```python
from build123d import *

# Parameters (mm, degrees)
Y_KSEKLIK_EKSTR_ZYON5_DEPTH      = 5
Y_KSEKLIK_EKSTR_ZYON5_DEPTH_BACK = 5
IZIM1_R                          = 37
IZIM1_R_2                        = 35.75
Y_KSEKLIK_EKSTR_ZYON6_DEPTH      = 3
Y_KSEKLIK_EKSTR_ZYON6_DEPTH_BACK = 3
IZIM1_13_R                       = 38.25
IZIM1_13_R_2                     = 37
Y_KSEKLIK_EKSTR_ZYON7_DEPTH      = 3
Y_KSEKLIK_EKSTR_ZYON7_DEPTH_BACK = 3
IZIM1_14_R                       = 1.5
Y_KSEKLIK_EKSTR_ZYON8_DEPTH      = 7
Y_KSEKLIK_EKSTR_ZYON8_DEPTH_BACK = 3


with BuildPart() as part:
    # Çizim1 → Yükseklik-Ekstrüzyon5 (new, two sides: drawn at the far end of the back side and taken through both)
    with BuildSketch(Plane.XY.offset(-Y_KSEKLIK_EKSTR_ZYON5_DEPTH_BACK)):
        Circle(IZIM1_R)
        Circle(IZIM1_R_2, mode=Mode.SUBTRACT)
    extrude(amount=Y_KSEKLIK_EKSTR_ZYON5_DEPTH + Y_KSEKLIK_EKSTR_ZYON5_DEPTH_BACK)

    # Çizim1<13> → Yükseklik-Ekstrüzyon6 (add, two sides: drawn at the far end of the back side and taken through both)
    with BuildSketch(Plane.XY.offset(-Y_KSEKLIK_EKSTR_ZYON6_DEPTH_BACK)):
        Circle(IZIM1_13_R)
        Circle(IZIM1_13_R_2, mode=Mode.SUBTRACT)
    extrude(amount=Y_KSEKLIK_EKSTR_ZYON6_DEPTH + Y_KSEKLIK_EKSTR_ZYON6_DEPTH_BACK)

    # Çizim1<14> → Yükseklik-Ekstrüzyon7 (add, two sides: drawn at the far end of the back side and taken through both)
    with BuildSketch(Plane.XY.offset(-Y_KSEKLIK_EKSTR_ZYON7_DEPTH_BACK)):
        with BuildLine():
            Line((0.352105211, 10.658426892), (0.352105211, 8.25))
            Line((0.352105211, 8.25), (0.352105211, 2.891667151))
            ThreePointArc((0.352105211, 2.891667151), (2.180757714, 1.931324101), (2.913025402, 0))
            ThreePointArc((2.913025402, 0), (-1.931880518, -2.180264813), (-0.350629391, 2.891846473))
            Line((-0.350629391, 2.891846473), (-0.347894744, 8.250178624))
            Line((-0.347894744, 8.250178624), (-0.346665593, 10.658605202))
            ThreePointArc((-0.346665593, 10.658605202), (-1.792646187, 11.069293289), (-2.984941087, 11.98469345))
            Line((-2.984941087, 11.98469345), (-14.607887345, 30.4259885))
            Line((-14.607887345, 30.4259885), (-14.847868654, 30.886461313))
            ThreePointArc((-14.847868654, 30.886461313), (-14.727142284, 32.060689053), (-13.92488883, 32.926584565))
            ThreePointArc((-13.92488883, 32.926584565), (-17.875, 30.960408185), (-21.552814278, 28.522599754))
            ThreePointArc((-21.552814278, 28.522599754), (-20.401800041, 28.78442387), (-19.324525803, 28.301862102))
            Line((-19.324525803, 28.301862102), (-19.045735303, 27.863795787))
            Line((-19.045735303, 27.863795787), (-8.886868167, 8.577081355))
            ThreePointArc((-8.886868167, 8.577081355), (-9.303777514, 5.496482546), (-11.800782256, 3.644761794))
            Line((-11.800782256, 3.644761794), (-33.653555768, 2.549643924))
            Line((-33.653555768, 2.549643924), (-34.19029782, 2.590308308))
            ThreePointArc((-34.19029782, 2.590308308), (-35.134400226, 3.283913251), (-35.477703108, 4.403984811))
            ThreePointArc((-35.477703108, 4.403984811), (-35.75, 0), (-35.477703108, -4.403984811))
            ThreePointArc((-35.477703108, -4.403984811), (-35.134400226, -3.283913251), (-34.19029782, -2.590308308))
            Line((-34.19029782, -2.590308308), (-33.653555768, -2.549643924))
            Line((-33.653555768, -2.549643924), (-11.802585687, -3.638917628))
            ThreePointArc((-11.802585687, -3.638917628), (-9.303458853, -5.492132995), (-8.888309481, -8.575587733))
            Line((-8.888309481, -8.575587733), (-19.045735303, -27.863795787))
            ThreePointArc((-19.045735303, -27.863795787), (-20.165883221, -28.700819486), (-21.552814278, -28.522599754))
            ThreePointArc((-21.552814278, -28.522599754), (-17.875, -30.960408185), (-13.92488883, -32.926584565))
            ThreePointArc((-13.92488883, -32.926584565), (-14.772697173, -31.814576902), (-14.607887345, -30.4259885))
            Line((-14.607887345, -30.4259885), (-2.984941087, -11.98469345))
            ThreePointArc((-2.984941087, -11.98469345), (0.002715908, -10.643228062), (2.991057136, -11.983168513))
            Line((2.991057136, -11.983168513), (14.663708375, -30.397995932))
            ThreePointArc((14.663708375, -30.397995932), (14.817986455, -31.815304786), (13.92488883, -32.926584565))
            ThreePointArc((13.92488883, -32.926584565), (17.875, -30.960408185), (21.552814278, -28.522599754))
            ThreePointArc((21.552814278, -28.522599754), (20.242255546, -28.76161283), (19.107217792, -28.064202809))
            Line((19.107217792, -28.064202809), (18.993975038, -27.89787469))
            Line((18.993975038, -27.89787469), (8.881942007, -8.582182507))
            ThreePointArc((8.881942007, -8.582182507), (9.294710999, -5.488602486), (11.804336715, -3.633233425))
            Line((11.804336715, -3.633233425), (33.657290889, -2.499854))
            Line((33.657290889, -2.499854), (33.849149755, -2.514104082))
            ThreePointArc((33.849149755, -2.514104082), (35.026532395, -3.146147751), (35.477703108, -4.403984811))
            ThreePointArc((35.477703108, -4.403984811), (35.681860841, -2.206197397), (35.75, 0))
            ThreePointArc((35.75, 0), (35.681860841, 2.206197397), (35.477703108, 4.403984811))
            ThreePointArc((35.477703108, 4.403984811), (35.026532395, 3.146147751), (33.849149755, 2.514104082))
            Line((33.849149755, 2.514104082), (33.657290889, 2.499854))
            Line((33.657290889, 2.499854), (11.803877394, 3.634725418))
            ThreePointArc((11.803877394, 3.634725418), (9.295867667, 5.489285508), (8.88302669, 8.581059795))
            Line((8.88302669, 8.581059795), (18.993975038, 27.89787469))
            Line((18.993975038, 27.89787469), (18.993582514, 27.898141932))
            ThreePointArc((18.993582514, 27.898141932), (20.143868947, 28.740405096), (21.552814278, 28.522599754))
            ThreePointArc((21.552814278, 28.522599754), (17.875, 30.960408185), (13.92488883, 32.926584565))
            ThreePointArc((13.92488883, 32.926584565), (14.817986455, 31.815304786), (14.663708375, 30.397995932))
            Line((14.663708375, 30.397995932), (14.663280674, 30.398202247))
            Line((14.663280674, 30.398202247), (2.991057136, 11.983168513))
            ThreePointArc((2.991057136, 11.983168513), (1.798295213, 11.068376963), (0.352105211, 10.658426892))
        make_face()
        with BuildLine():
            ThreePointArc((-15.330091906, -28.374268836), (-15.633406502, -28.599064993), (-16.007432074, -28.547704226))
            Line((-16.007432074, -28.547704226), (-16.719321042, -28.136694938))
            ThreePointArc((-16.719321042, -28.136694938), (-16.950813558, -27.838459675), (-16.907791673, -27.46338345))
            Line((-16.907791673, -27.46338345), (-8.752791972, -12.583042517))
            ThreePointArc((-8.752791972, -12.583042517), (-8.44909878, -12.341848787), (-8.064321341, -12.3903286))
            Line((-8.064321341, -12.3903286), (-6.698178659, -13.179071446))
            ThreePointArc((-6.698178659, -13.179071446), (-6.463805189, -13.488058576), (-6.52083849, -13.87166146))
            Line((-6.52083849, -13.87166146), (-15.330091906, -28.374268836))
        make_face(mode=Mode.SUBTRACT)
        with Locations((-4.7625, -8.25)):
            Circle(IZIM1_14_R, mode=Mode.SUBTRACT)
        with BuildLine():
            Line((16.719321042, -28.136694938), (16.007432074, -28.547704226))
            ThreePointArc((16.007432074, -28.547704226), (15.633406502, -28.599064993), (15.330091906, -28.374268836))
            Line((15.330091906, -28.374268836), (6.52083849, -13.87166146))
            ThreePointArc((6.52083849, -13.87166146), (6.463805189, -13.488058576), (6.698178659, -13.179071446))
            Line((6.698178659, -13.179071446), (8.064321341, -12.3903286))
            ThreePointArc((8.064321341, -12.3903286), (8.44909878, -12.341848787), (8.752791972, -12.583042517))
            Line((8.752791972, -12.583042517), (16.907791673, -27.46338345))
            ThreePointArc((16.907791673, -27.46338345), (16.950813558, -27.838459675), (16.719321042, -28.136694938))
        make_face(mode=Mode.SUBTRACT)
        with Locations((4.7625, -8.25)):
            Circle(IZIM1_14_R, mode=Mode.SUBTRACT)
        with BuildLine():
            Line((-32.726753116, -0.411009288), (-32.726753116, 0.411009288))
            ThreePointArc((-32.726753116, 0.411009288), (-32.584220059, 0.760605318), (-32.237883578, 0.910885385))
            Line((-32.237883578, 0.910885385), (-15.273630462, 1.288618943))
            ThreePointArc((-15.273630462, 1.288618943), (-14.91290397, 1.146209789), (-14.7625, 0.788742846))
            Line((-14.7625, 0.788742846), (-14.7625, -0.788742846))
            ThreePointArc((-14.7625, -0.788742846), (-14.91290397, -1.146209789), (-15.273630462, -1.288618943))
            Line((-15.273630462, -1.288618943), (-32.237883578, -0.910885385))
            ThreePointArc((-32.237883578, -0.910885385), (-32.584220059, -0.760605318), (-32.726753116, -0.411009288))
        make_face(mode=Mode.SUBTRACT)
        with Locations((-4.7625, 0)):
            Circle(IZIM1_14_R, mode=Mode.SUBTRACT)
        with Locations((-4.7625, 8.25)):
            Circle(IZIM1_14_R, mode=Mode.SUBTRACT)
        with BuildLine():
            ThreePointArc((-6.52083849, 13.87166146), (-6.463805189, 13.488058576), (-6.698178659, 13.179071446))
            Line((-6.698178659, 13.179071446), (-8.064321341, 12.3903286))
            ThreePointArc((-8.064321341, 12.3903286), (-8.44909878, 12.341848787), (-8.752791972, 12.583042517))
            Line((-8.752791972, 12.583042517), (-16.907791673, 27.46338345))
            ThreePointArc((-16.907791673, 27.46338345), (-16.950813558, 27.838459675), (-16.719321042, 28.136694938))
            Line((-16.719321042, 28.136694938), (-16.007432074, 28.547704226))
            ThreePointArc((-16.007432074, 28.547704226), (-15.633406502, 28.599064993), (-15.330091906, 28.374268836))
            Line((-15.330091906, 28.374268836), (-6.52083849, 13.87166146))
        make_face(mode=Mode.SUBTRACT)
        with Locations((4.7625, 0)):
            Circle(IZIM1_14_R, mode=Mode.SUBTRACT)
        with Locations((4.7625, 8.25)):
            Circle(IZIM1_14_R, mode=Mode.SUBTRACT)
        with BuildLine():
            ThreePointArc((32.237883578, 0.910885385), (32.584220059, 0.760605318), (32.726753116, 0.411009288))
            Line((32.726753116, 0.411009288), (32.726753116, -0.411009288))
            ThreePointArc((32.726753116, -0.411009288), (32.584220059, -0.760605318), (32.237883578, -0.910885385))
            Line((32.237883578, -0.910885385), (15.273630462, -1.288618943))
            ThreePointArc((15.273630462, -1.288618943), (14.91290397, -1.146209789), (14.7625, -0.788742846))
            Line((14.7625, -0.788742846), (14.7625, 0.788742846))
            ThreePointArc((14.7625, 0.788742846), (14.91290397, 1.146209789), (15.273630462, 1.288618943))
            Line((15.273630462, 1.288618943), (32.237883578, 0.910885385))
        make_face(mode=Mode.SUBTRACT)
        with BuildLine():
            Line((8.064321341, 12.3903286), (6.698178659, 13.179071446))
            ThreePointArc((6.698178659, 13.179071446), (6.463805189, 13.488058576), (6.52083849, 13.87166146))
            Line((6.52083849, 13.87166146), (15.330091906, 28.374268836))
            ThreePointArc((15.330091906, 28.374268836), (15.633406502, 28.599064993), (16.007432074, 28.547704226))
            Line((16.007432074, 28.547704226), (16.719321042, 28.136694938))
            ThreePointArc((16.719321042, 28.136694938), (16.950813558, 27.838459675), (16.907791673, 27.46338345))
            Line((16.907791673, 27.46338345), (8.752791972, 12.583042517))
            ThreePointArc((8.752791972, 12.583042517), (8.44909878, 12.341848787), (8.064321341, 12.3903286))
        make_face(mode=Mode.SUBTRACT)
    extrude(amount=Y_KSEKLIK_EKSTR_ZYON7_DEPTH + Y_KSEKLIK_EKSTR_ZYON7_DEPTH_BACK)

    # Çizim1<17> → Yükseklik-Ekstrüzyon8 (add, two sides: drawn at the far end of the back side and taken through both)
    with BuildSketch(Plane.XY.offset(-Y_KSEKLIK_EKSTR_ZYON8_DEPTH_BACK)):
        with BuildLine():
            ThreePointArc((2.913025402, 0), (2.180757714, 1.931324101), (0.352105211, 2.891667151))
            Line((0.352105211, 2.891667151), (0.352105211, 1.458088447))
            ThreePointArc((0.352105211, 1.458088447), (1.387985779, 0.568766629), (1.274033112, -0.791732044))
            Line((1.274033112, -0.791732044), (-1.274033112, -0.791732044))
            ThreePointArc((-1.274033112, -0.791732044), (-1.387840597, 0.569120792), (-0.351361024, 1.458267956))
            Line((-0.351361024, 1.458267956), (-0.350629391, 2.891846473))
            ThreePointArc((-0.350629391, 2.891846473), (-1.931880518, -2.180264813), (2.913025402, 0))
        make_face()
    extrude(amount=Y_KSEKLIK_EKSTR_ZYON8_DEPTH + Y_KSEKLIK_EKSTR_ZYON8_DEPTH_BACK)


solid = part.part
```
Check sheet for the modelled part. Datum: model origin and axes. Units: mm. Round coordinates to 2 decimals unless told otherwise and drop trailing zeros.
1) Go/stop test with flat-tipped pins: pin 1 Ø8 at (x, y) = (17, -19.5) entering from -Z; pin 2 Ø0.8 at (x, z) = (-0.5, 1.5) entering from +Y; pin 3 Ø1 at (y, z) = (2.5, -2.5) entering from +X. Record where each tip stops, or that it passes through.
2) Section check A-A (x = 20.5). Give the number of separate pieces and of enclosed holes in the cut face, and give its area (3 significant figures).
3) Scan lines: line 1 (X direction, y = -9, z = -0.5); line 2 (Y direction, x = 25, z = 2.25); line 3 (Z direction, x = 6.5, y = 0). Record each from-to range of solid material in increasing order.
4) Mould release check, pull along Y, two halves, no side actions. Record for faces 1 (the cylindrical face through (-9.3, -5.5, 0)), 2 (the flat face through (0, -1, 7)), 3 (the cylindrical face through (-30.354, -23.275, -0.042)): +Y half, -Y half, draft (parallel to the pull), parting line (faces both ways), or undercut.
Result:
1. pin 1: stops at z = -3
1. pin 2: stops at y = 38.25
1. pin 3: stops at x = 38.2
2. separate pieces: 4
2. enclosed holes: 0
2. area: 78.2 mm2
3. line 1: x = -37.18 to -34.6, -9.11 to -6.06, -3.46 to 3.46, 6.06 to 9.1, 34.6 to 37.18
3. line 2: y = -28.95 to -25.56, -2.95 to -1.07, 1.07 to 2.95, 25.56 to 28.95
3. line 3: z = -3 to 3
4. face 1: undercut
4. face 2: draft
4. face 3: parting line
